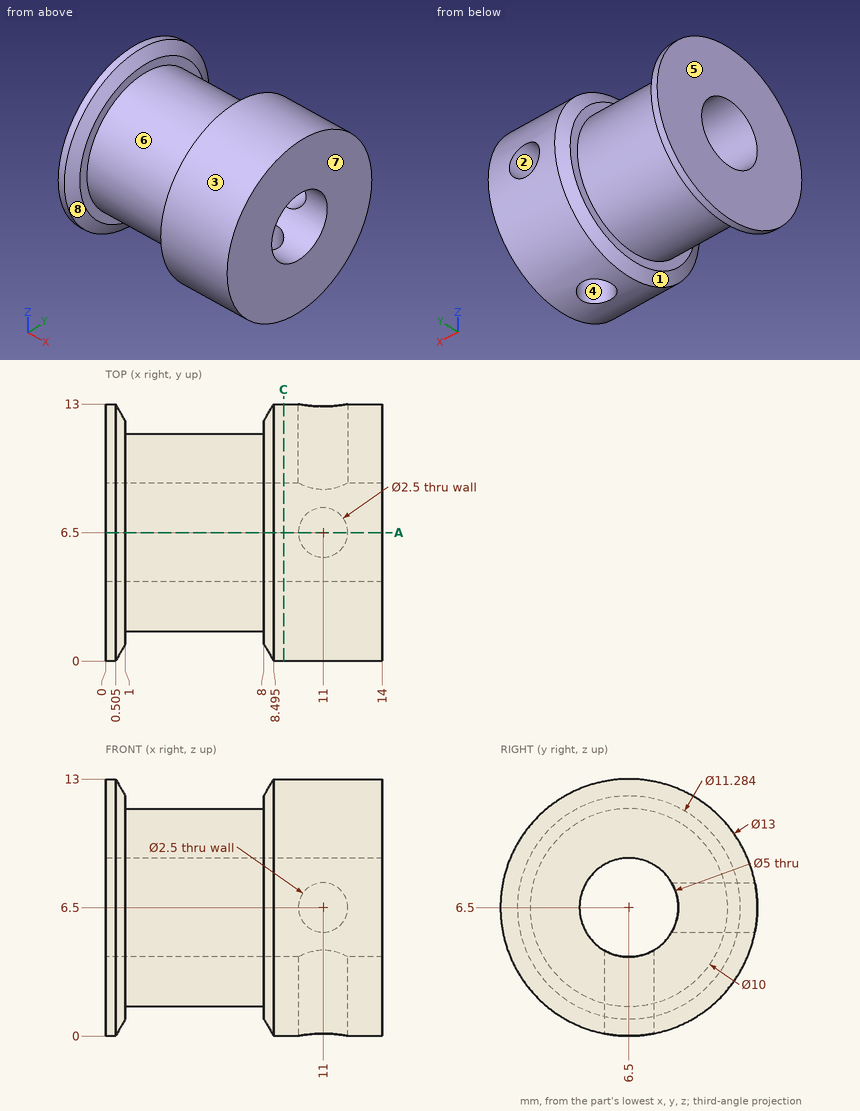
Job drawing, mm, ordinate dimensions from the low corner. One solid piece. A direction names the side the tool comes from. Coordinates: 2 decimals unless noted, no trailing zeros. Order: outer loops, then holes, each group sorted by start corner. A loop starts at its lowest first (then second) coordinate and runs counter-clockwise, first axis right, second up. Notation, with made-up numbers: (-4.75, 39.25) -> (1.25, 39.25) arc R14 cw to (1.25, 50.25) -> close; hole circle Ø1 at (25.5, 51.25). An arc over 180 degrees is marked (long way). Put each result on its own line as item: value. Start each with the question number.
(1) Pin check, flat tips, straight feed: pin 1 Ø6 at (x, z) = (7.5, 3.5) entering from +Y; pin 2 Ø1.5 at (x, z) = (12, 9.5) entering from +Y. Stop position of each tip, or through.
(2) Band-saw the part on A-A (y = 6.5). Count the separate pieces of the cut face and the enclosed holes in it.
(3) Band-saw the part on C-C (x = 9). Give the cut face in (y, z).
(4) Mould opens along X. For the marked faces 5, 6, 7 and 8 say: pulls with the +X half, pulls with the -X half, needs draft (parallel to the pull), parting line crosses it, or undercut.
(5) Which spindle directions (+Z, -Z, +X, -X, +Y, -Y) get a long thin tool onto all of the face, cutting with end or side? Do the marked faces 1, 2, 3 and 4. Say none if no direction does.
(6) Probe line 1 along X through (y, z) = (1.75, 3.5); line 2 along Z through (x, y) = (3, 7.75) (1 decimal); line 3 along Z through (x, y) = (11, 11.6). List the from-to ranges inside material, lowest first. Write a range as [from, to].
Determined:
1. pin 1: stops at y = 13
1. pin 2: stops at y = 12.6
2. separate pieces: 3
2. enclosed holes: 0
3. outline: circle Ø13 at (6.5, 6.5); hole circle Ø5 at (6.5, 6.5)
4. face 5: pulls with the -X half
4. face 6: undercut
4. face 7: pulls with the +X half
4. face 8: undercut
5. face 1: none
5. face 2: +Y
5. face 3: +X, -X
5. face 4: -Z
6. line 1: x = [0, 1], [8, 14]
6. line 2: z = [1.7, 4.3], [8.7, 11.3]
6. line 3: z = [2.47, 5.25], [7.75, 10.53]
